The drawing under review shows one solid part. Ordinate dimensions are in mm from its lowest x, y, z. Give positions to 0.01 mm unless a question says otherwise; leave off trailing zeros. Write each loop counter-clockwise with the first axis right and the second up, starting at its lowest first coordinate (ties: lowest second). Pieces come first, ordered by that corner, then holes. Notation, with made-up numbers: M 37.25,-28.75 L 86.25,-28.75 A23 cw 86.25,0.25 Z; hole C -35,5 d8. An arc over 180 degrees is marked long. One line per item, written item: value. Start each with the question number.
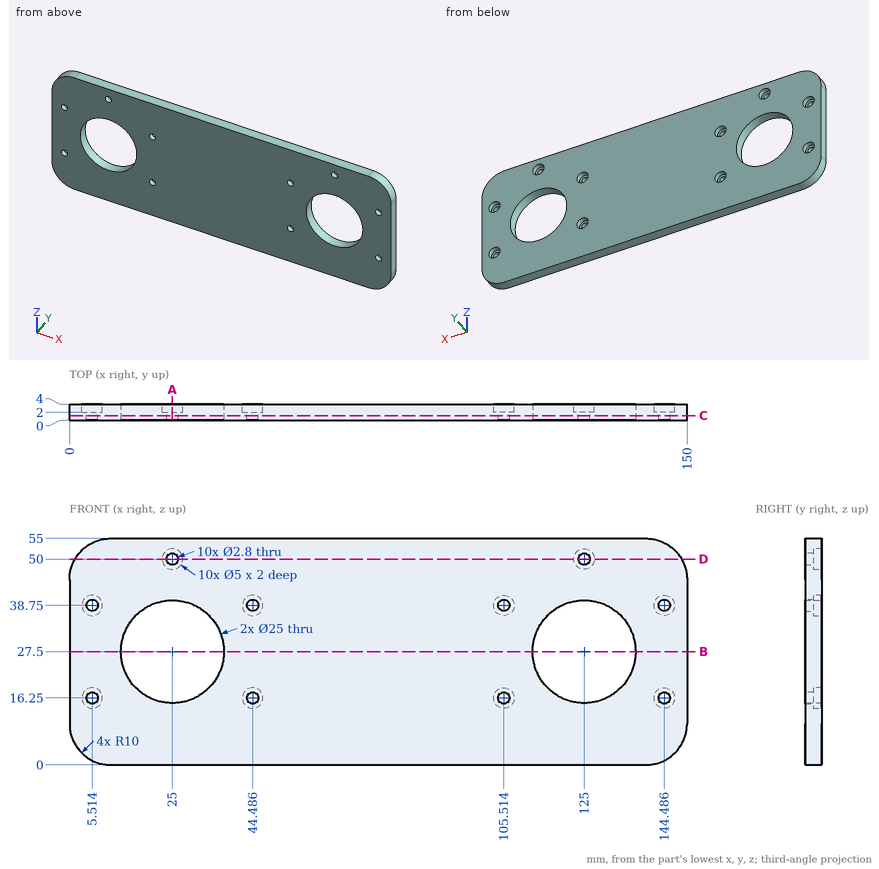
Q1. Take a section at A-A, the plane x = 25. Give the boundary of the cut face in (y, z).
Q2. For P1, Ø3, axis at x = 5.51, z = 16.25, coming from the +Y side, flat-tipped, find the tip position at first contact; note if it passes through.
Q3. Take a section at D-D, the plane z = 50. Give the boundary of the cut face in (x, y), then the cut area to 3 significant figures.
Q4. Take a section at B-B, the plane z = 27.5. Give the boundary of the cut face in (x, y), then the cut area to 3 significant figures.
Q5. Wall thickness on line 1 (X direction, y = 0.2, z = 31); line 2 (X direction, y = 0.95, z = 50); line 3 (Z direction, x = 19.5, y = 3.35) (1 decimal): over which ranges is each line inside the solid? List them lowest first. Write a range as from..to.
Q6. Take a section at C-C, the plane y = 1.2. State how many separate pieces and enclosed holes the cut face has, then the cut area to 3 significant figures.
Results list:
1. outline: M 0,0 L 4,0 L 4,15 L 0,15 Z; M 0,40 L 4,40 L 4,47.5 L 2,47.5 L 2,48.6 L 0,48.6 Z; M 0,51.4 L 2,51.4 L 2,52.5 L 4,52.5 L 4,55 L 0,55 Z
2. P1: stops at y = 2
3. outline: M 1.34,0 L 23.6,0 L 23.6,2 L 22.5,2 L 22.5,4 L 1.34,4 Z; M 26.4,0 L 123.6,0 L 123.6,2 L 122.5,2 L 122.5,4 L 27.5,4 L 27.5,2 L 26.4,2 Z; M 126.4,0 L 148.66,0 L 148.66,4 L 127.5,4 L 127.5,2 L 126.4,2 Z
3. area: 558 mm^2
4. outline: M 0,0 L 12.5,0 L 12.5,4 L 0,4 Z; M 37.5,0 L 112.5,0 L 112.5,4 L 37.5,4 Z; M 137.5,0 L 150,0 L 150,4 L 137.5,4 Z
4. area: 400 mm^2
5. line 1: x = 0..13, 37..113, 137..150
5. line 2: x = 1.34..23.6, 26.4..123.6, 126.4..148.66
5. line 3: z = 0..16.3, 38.7..55
6. separate pieces: 1
6. enclosed holes: 12
6. area: 7,120 mm^2
